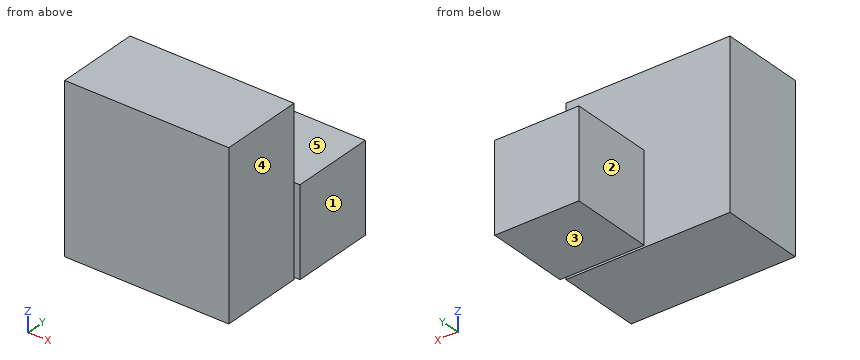
```python
from build123d import *

# Parameters (mm, degrees)
F0_W     = 39
F0_H     = 39
F1_DEPTH = 20
F3_DEPTH = 20


with BuildPart() as f1:
    # F0 (on Front) → F1 (new body)
    with BuildSketch(Plane.XZ):
        with Locations((-0.900001, -1.994445)):
            Rectangle(F0_W, F0_H)
    extrude(amount=F1_DEPTH)

    # F2 (on Right) → F3 (join)
    with BuildSketch(Plane.YZ):
        Polygon((20, 0), (0, 0), (0, -18.648019), (0, -21), (20, -21), align=None)
    extrude(amount=F3_DEPTH)


solid = f1.part
```
The model under review builds one solid part; all positions refer to its coordinate system, in mm. Face numbers are marked on the shaded views. A direction names the side the tool comes from. Coordinates: 2 decimals unless noted, no trailing zeros. Order: outer loops, then holes, each group sorted by start corner. A loop starts at its lowest first (then second) coordinate and runs counter-clockwise, first axis right, second up. Notation, with made-up numbers: (-14, 14.5) -> (13, 14.5) arc R21 ccw to (13, 41.5) -> close; hole circle Ø3 at (43.25, -6.5). An arc over 180 degrees is marked (long way). Answer in a Markdown table with one row per item. Add a question column.
Item 1: We need section C-C on y = 14. Write out the cut boundary in (x, z).
Item 2: Machinability: for the marked faces 1, 2, 3, 4 and 5, which of the approach directions +Z, -Z, +X, -X, +Y, -Y give a long, thin tool a straight path to every point of the face, cutting with its end or side? Answer none if there is none.
Item 3: We need section D-D on y = -15.5. Write out the cut boundary in (x, z), plus the area to 3 significant figures.
Item 4: Clearance check with flat-ended pins moving along their axes: pin 1 (4 mm diameter, centred on x = 10.5, y = 13, fed in from +Z); pin 2 (10 mm diameter, centred on y = 9, z = -9, fed in from -X); pin 3 (1.1 mm diameter, centred on x = 19.5, z = -6, fed in from -Y). State where each tip first meets the part, or that it passes through.
Item 5: To check wall thickness, follow probe 1 along X at (y, z) = (-16, 11); probe 2 along Z at (x, y) = (18.5, 12.5); probe 3 along Y at (x, z) = (-12.5, 15.5). State the ranges of each line that lie inside material, in increasing order.
Item 6: We need section A-A on x = 3.5. Write out the cut boundary in (y, z).
Item 7: We need section B-B on z = -16.5. Write out the cut boundary in (x, y).
Final values:
| question | item | result |
|---|---|---|
| 1 | outline | (0, -21) -> (20, -21) -> (20, 0) -> (0, 0) -> close |
| 2 | face 1 | +Z, -Z, +X, +Y, -Y |
| 2 | face 2 | +Z, -Z, -X, +Y |
| 2 | face 3 | -Z, +X, -X, +Y |
| 2 | face 4 | +Z, -Z, +X, -Y |
| 2 | face 5 | +Z, +X, -X, +Y |
| 3 | outline | (-20.4, -21.49) -> (18.6, -21.49) -> (18.6, 17.51) -> (-20.4, 17.51) -> close |
| 3 | area | 1,520 mm2 |
| 4 | pin 1 | stops at z = 0 |
| 4 | pin 2 | stops at x = 0 |
| 4 | pin 3 | stops at y = 0 |
| 5 | probe 1 | x = -20.4 to 18.6 |
| 5 | probe 2 | z = -21 to 0 |
| 5 | probe 3 | y = -20 to 0 |
| 6 | outline | (-20, -21.49) -> (0, -21.49) -> (0, -21) -> (20, -21) -> (20, 0) -> (0, 0) -> (0, 17.51) -> (-20, 17.51) -> close |
| 7 | outline | (-20.4, -20) -> (18.6, -20) -> (18.6, 0) -> (20, 0) -> (20, 20) -> (0, 20) -> (0, 0) -> (-20.4, 0) -> close |
